Read the model definition and answer for the solid it produces. Units are mm, in the model's axes. A direction names the side the tool comes from. Round coordinates to 2 decimals unless told otherwise and drop trailing zeros. Order: outer loops, then holes, each group sorted by start corner. A loop starts at its lowest first (then second) coordinate and runs counter-clockwise, first axis right, second up. Notation, with made-up numbers: (37, 65.25) -> (61, 65.25) arc R21 ccw to (61, 73.25) -> close; hole circle Ø9 at (64, 30). An arc over 180 degrees is marked (long way). Answer as a JSON object with one key per item and string values. Group by question number.
Item 1: Section C-C, the plane x = 2 is taken. Write down the section's boundary in (y, z), plus the area to 3 significant figures.
Item 2: Section D-D, the plane y = 9 is taken. Write down the section's boundary in (x, z).
Item 3: For faces 4 (the cylindrical face through (0, 18, 9)), 5 (the flat face through (-2, 20, 20)), 6 (the cylindrical face through (5.302, 5.085, -15.832)), 7 (the cylindrical face through (-17.01, 34.42, -1.11)), determine the directions among +Z, -Z, +X, -X, +Y, -Y from which every point of the face is accessible in a straight line to the end or side of a thin tool.
Item 4: Section B-B, the plane z = 7 is taken. Write down the section's boundary in (x, y), plus the area to 3 significant figures.
Item 5: Given P1, Ø2.5, axis at x = -3, z = 0, coming from the +Y side; P2, Ø10, axis at x = -5.5, y = 34, coming from the -Z side; P3, Ø8, axis at y = 19.5, z = -10.5, coming from the -X side, each flat-ended and moving along its own axis, determine where each tip first touches the part or whether it passes through.
Item 6: Section A-A, the plane y = 34.5 is taken. Write down the section's boundary in (x, z), plus the area to 3 significant figures.
Item 7: The mould has two halves that part along Z. Classify faces 1 (the flat face through (4, 15, -28)), 2 (the cylindrical face through (-1.536, 34.423, -0.325)), 3 (the flat face through (-9, 40, 3)): pulls with the +Z half, pulls with the -Z half, needs draft (parallel to the pull), parting line crosses it, or undercut.
Item 8: Consider probe 1 along X at (y, z) = (33, 0); probe 2 along Z at (x, y) = (-16, 35); probe 3 along Z at (x, y) = (-3, 37). Determine where each line is inside the solid, lowest interval first. Write a range as from..to.
Autodesk Inventor part; units mm, degrees
ref_plane "YZ Plane" through (0, 0, 0) normal (1, 0, 0) x (0, 1, 0)
ref_plane "XZ Plane" through (0, 0, 0) normal (0, 1, 0) x (-1, 0, 0)
ref_plane "XY Plane" through (0, 0, 0) normal (0, 0, 1) x (1, 0, 0)
sketch "Sketch1" plane through (0, 0, 0) normal (0, 1, 0) x (-1, 0, 0)
  line L0 (-20, 4) -> (20, 4)
  line L1 (20, 4) -> (20, -4)
  line L2 (20, -4) -> (-20, -4)
  line L3 (-20, -4) -> (-20, 4)
  line L4 (-20, 4) -> (20, -4) construction
  line L5 (20, 4) -> (-20, -4) construction
  line L6 (20, -4) -> (12, -4)
  line L7 (12, -4) -> (12, 36)
  line L8 (12, 36) -> (20, 36)
  line L9 (20, 36) -> (20, -4)
  point P0 (0, 0)
  point P1 (12, 4)
  dimension "d0" = 40
  dimension "d1" = 8
  dimension "d2" = 8
  dimension "d3" = 40
extrude "Extrusion1" add sketch "Sketch1" along normal blind 40
sketch "Sketch2" plane through (0, 40, 0) normal (0, 1, 0) x (1, 0, 0)
  circle A0 centre (8, 0) radius 2.5
  circle A1 centre (-3, 0) radius 2.5
  circle A2 centre (-16, 0) radius 2.5
  circle A3 centre (-16, -23.5) radius 2.5
  line L0 (20, -4) -> (20, 4)
  line L1 (-20, -36) -> (-12, -36)
  point P0 (0, 0)
  point P1 (-16, -36)
  point P2 (-16, -36)
  point P3 (20, 0)
  point P4 (-16, -36)
  point P5 (20, 0)
  dimension "d6" = 5
  dimension "d7" = 5
  dimension "d8" = 5
  dimension "d9" = 5
  dimension "d10" = 12
  dimension "d21" = 12.5
  dimension "d22" = 23
hole "Hole1" at (-16, 40, 23.5) at (-16, 40, 0) at (-3, 40, 0) at (8, 40, 0) direction (0, -1, 0) diameter 3 depth 11 tip angle 118
sketch "Sketch3" plane through (-12, 0, 36) normal (1, 0, 0) x (0, 0, -1)
  circle A0 centre (16, 20) radius 5
  line L0 (0, 0) -> (0, 40)
  point P0 (36, 0)
  dimension "d23" = 10
  dimension "d31" = 16
extrude "Extrusion2" add sketch "Sketch3" along normal blind 10
sketch "Sketch4" plane through (-12, 0, 4) normal (0, 0, 1) x (1, 0, 0)
  circle A0 centre (16, 15) radius 5
  line L0 (0, 0) -> (32, 0)
  line L1 (32, 0) -> (32, 40)
  point P0 (12, 0)
  dimension "d26" = 10
  dimension "d27" = 15
  dimension "d28" = 16
extrude "Extrusion3" add sketch "Sketch4" along normal blind 10
sketch "Sketch5" plane through (20, 0, -4) normal (0, 0, -1) x (-1, 0, 0)
  circle A0 centre (16, 15) radius 5
  circle A1 centre (16, 15) radius 10
  point P0 (20, 0)
  dimension "d32" = 20
extrude "Extrusion4" add sketch "Sketch5" along normal blind 24 contours A0 | A1
equation "\"d19\" = d11"
properties part number "Non-ThorLabs Galvo"
Values found:
{
 "1": {"outline": "(0, -4) -> (5.2, -4) -> (5.2, -28) -> (24.8, -28) -> (24.8, -4) -> (40, -4) -> (40, 4) -> (19.58, 4) -> (19.58, 14) -> (10.42, 14) -> (10.42, 4) -> (0, 4) -> close", "area": "882 mm2"},
 "2": {"outline": "(-20, -4) -> (-4, -4) -> (-4, -28) -> (12, -28) -> (12, -4) -> (20, -4) -> (20, 4) -> (-12, 4) -> (-12, 36) -> (-20, 36) -> close"},
 "3": {"face 4": "+Z", "face 5": "+Z, +X, +Y, -Y", "face 6": "-Z", "face 7": "+Y"},
 "4": {"outline": "(-20, 0) -> (-12, 0) -> (-12, 40) -> (-20, 40) -> close; circle Ø10 at (4, 15)", "area": "399 mm2"},
 "5": {"P1": "y = 28.85", "P2": "z = -4", "P3": "x = -5.99"},
 "6": {"outline": "(-20, -4) -> (20, -4) -> (20, 4) -> (-12, 4) -> (-12, 36) -> (-20, 36) -> close; hole circle Ø3 at (-16, 0); hole circle Ø3 at (-16, 23.5); hole circle Ø3 at (-3, 0); hole circle Ø3 at (8, 0)", "area": "548 mm2"},
 "7": {"face 1": "pulls with the -Z half", "face 2": "undercut", "face 3": "needs draft"},
 "8": {"probe 1": "-20..-17.5, -14.5..-4.5, -1.5..6.5, 9.5..20", "probe 2": "-4..-1.5, 1.5..22, 25..36", "probe 3": "-4..-1.5, 1.5..4"}
}
